```python
from build123d import *

# Parameters (mm, degrees)
F1_DEPTH     = 3.175
F2_T1_DEPTH  = 39.0408928639
F2_T3_DEPTH  = 42.1701237591
F2_T5_DEPTH  = 62.58572165
F2_T7_DEPTH  = 42.1701213881
F2_T9_DEPTH  = 42.7652991577
F2_T11_DEPTH = 62.8914365267
F2_T13_DEPTH = 42.7652991577


# Not quite as in the source:
# - a fillet or chamfer that OpenCascade refuses, or shapes differently, is made with other operations: its cross-section is extruded or revolved along the edge and cut away or added


with BuildPart() as f1:
    # F0 (on Top) → F1 (new body)
    with BuildSketch(Plane.XY):
        Polygon((28.8131255029, 6.9092694693), (18.2287094494, 18.963740563), (-18.2287130429, 18.963740563), (-28.8131255029, 6.9092694693), (-28.8131255029, -6.0033242369), (-18.3815686845, -18.963740563), (18.3815686845, -18.963740563), (28.8131255029, -6.0033242369), align=None)
    extrude(amount=F1_DEPTH)

    # F2: chamfer of 5.08 on 8 edges, made by hand

    # F2_s2 → F2_t1 (cut)
    with BuildSketch(Plane.XZ.offset(-19.9734190482)):
        Polygon((28.8131255029, -1.905), (23.7331255029, 3.175), (28.8131255029, 3.175), align=None)
        Polygon((-28.8131255029, -1.905), (-23.7331255029, 3.175), (-28.8131255029, 3.175), align=None)
    extrude(amount=F2_T1_DEPTH, mode=Mode.SUBTRACT)

    # F2_s4 → F2_t3 (cut)
    with BuildSketch(Plane(origin=(17.7375583227, -20.2011034897, 0), x_dir=(0, 0, 1), z_dir=(-0.6598012581, 0.7514401506, 0))):
        Polygon((-1.905, 26.210084054), (3.175, 21.130084054), (3.175, 26.210084054), align=None)
    extrude(amount=F2_T3_DEPTH, mode=Mode.SUBTRACT)

    # F2_s6 → F2_t5 (cut)
    with BuildSketch(Plane.YZ.offset(-31.2928626217)):
        Polygon((18.963740563, -1.905), (13.883740563, 3.175), (18.963740563, 3.175), align=None)
    extrude(amount=F2_T5_DEPTH, mode=Mode.SUBTRACT)

    # F2_s8 → F2_t7 (cut)
    with BuildSketch(Plane(origin=(10.0863417988, 11.4872238883, 0), x_dir=(0, 0, 1), z_dir=(-0.6598011316, -0.7514402616, 0))):
        Polygon((-1.905, 26.2100863801), (3.175, 21.1300863801), (3.175, 26.2100863801), align=None)
    extrude(amount=F2_T7_DEPTH, mode=Mode.SUBTRACT)

    # F2_s10 → F2_t9 (cut)
    with BuildSketch(Plane(origin=(-16.5866539058, 20.6076565386, 0), x_dir=(0, 0, 1), z_dir=(0.627009486, -0.7790116202, 0))):
        Polygon((-1.905, 26.2099008264), (3.175, 21.1299008264), (3.175, 26.2099008264), align=None)
    extrude(amount=F2_T9_DEPTH, mode=Mode.SUBTRACT)

    # F2_s12 → F2_t11 (cut)
    with BuildSketch(Plane.YZ.offset(-31.4457182634)):
        Polygon((-18.963740563, -1.905), (-13.883740563, 3.175), (-18.963740563, 3.175), align=None)
    extrude(amount=F2_T11_DEPTH, mode=Mode.SUBTRACT)

    # F2_s14 → F2_t13 (cut)
    with BuildSketch(Plane(origin=(-10.2275943371, -12.7070084487, 0), x_dir=(0, 0, 1), z_dir=(0.627009486, 0.7790116202, 0))):
        Polygon((-1.905, 26.2099008264), (3.175, 21.1299008264), (3.175, 26.2099008264), align=None)
    extrude(amount=F2_T13_DEPTH, mode=Mode.SUBTRACT)


solid = f1.part
```
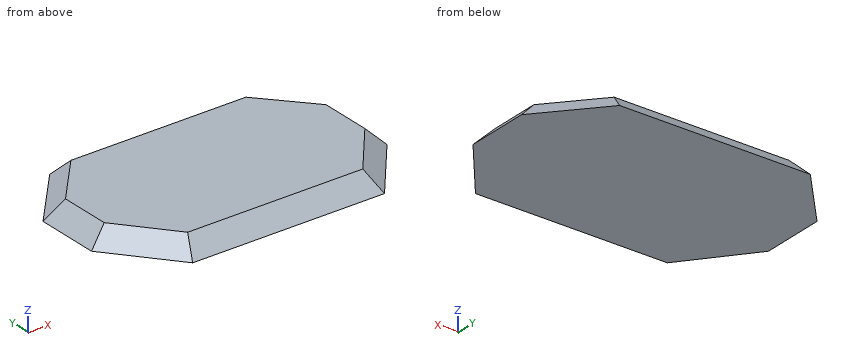
Work out the finished part from the listing and answer in its coordinate system (mm). Give positions to 0.01 mm unless a question says otherwise; leave off trailing zeros. Loops run counter-clockwise (first coordinate to the right, second up) from the corner with the lowest first, then second, coordinate; pieces in that order, holes last. Notation, with made-up numbers: (-17, 41) -> (23, 41) arc R11 ccw to (23, 60) -> close; hole circle Ø8 at (25, -16.75). An arc over 180 degrees is marked (long way). One line per question, with ' | ' between items. Start each with the question number.
1) Straight lines are drawn through the part: L1, parallel to X at y = -9, z = 2.05; L2, parallel to Z at x = 11.5, y = -14.5; L3, parallel to X at y = -5, z = 2.7. For each, find the intervals that lie inside material, in ascending order.
2) Section A-A, the plane z = 2.15 is taken. Determine the outline of the cut face in (x, y), then the cut area to 3 significant figures.
3) Section C-C, the plane y = -0.5 is taken. Determine the outline of the cut face in (x, z) (3 decimals).
4) Section B-B, the plane x = 11 is taken. Determine the outline of the cut face in (y, z) (3 decimals).
Resolved:
1) L1: -21.32 to 21.32 | L2: 0 to 2.56 | L3: -23.71 to 23.71
2) outline: (-24.76, -4.57) -> (-16.44, -14.91) -> (16.44, -14.91) -> (24.76, -4.57) -> (24.76, 5.38) -> (16.39, 14.91) -> (-16.39, 14.91) -> (-24.76, 5.38) -> close | area: 1,310 mm2
3) outline: (-26.908, 0) -> (26.908, 0) -> (23.733, 3.175) -> (-23.733, 3.175) -> close
4) outline: (-17.059, 0) -> (17.059, 0) -> (13.884, 3.175) -> (-13.884, 3.175) -> close
